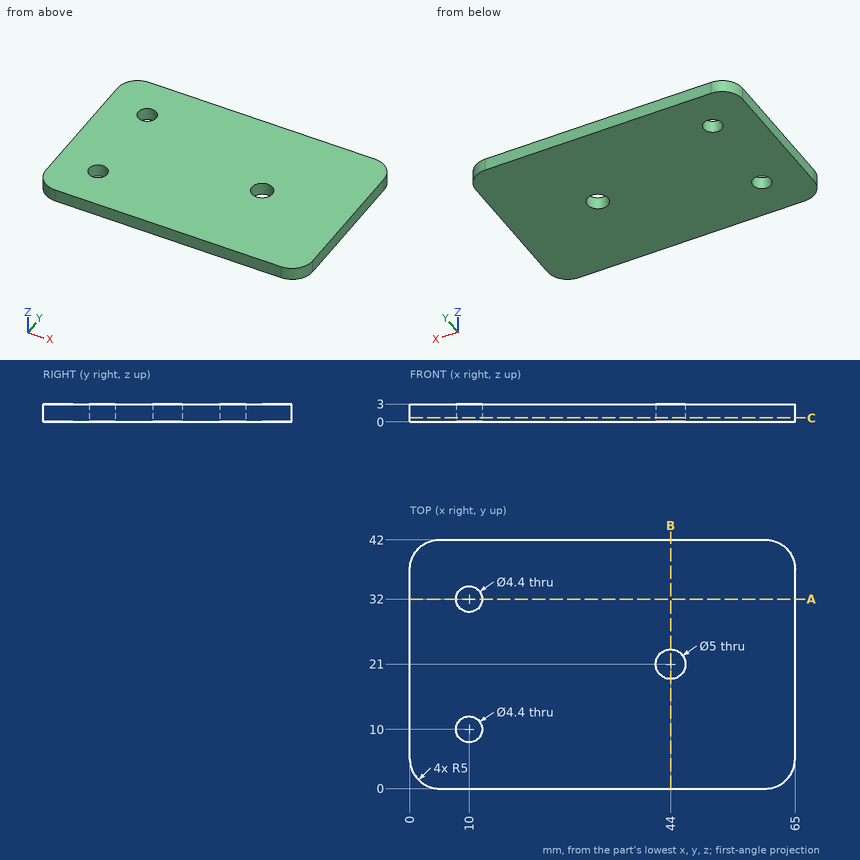
The figure shows three views and two pictorial views of one solid part (mm, origin at its lowest corner). Answer the questions. Give positions to 0.01 mm unless a question says otherwise; leave off trailing zeros. Loops run counter-clockwise (first coordinate to the right, second up) from the corner with the lowest first, then second, coordinate; pieces in that order, holes last. Notation, with made-up numbers: (64.25, 14) -> (87.25, 14) arc R31 ccw to (87.25, 38) -> close; hole circle Ø5 at (-2, 1). An arc over 180 degrees is marked (long way). Put each result on its own line as item: value. Start each with the question number.
Item 1: The part is cut by section C-C (z = 0.65). Give the vertices of the cut face in (x, y), then the cut area to 3 significant figures.
Item 2: The part is cut by section B-B (x = 44). Give the vertices of the cut face in (y, z).
Item 3: Find the intervals of material crossed by L1, parallel to Y at x = 10, z = 1.8; L2, parallel to X at y = 31, z = 2.65; L3, parallel to X at y = 23, z = 0.8, in increasing order. Write a range as [from, to].
Item 4: The part is cut by section A-A (y = 32). Give the vertices of the cut face in (x, z), then the cut area to 3 significant figures.
Answers below:
1. outline: (0, 5) arc R5 ccw to (5, 0) -> (60, 0) arc R5 ccw to (65, 5) -> (65, 37) arc R5 ccw to (60, 42) -> (5, 42) arc R5 ccw to (0, 37) -> close; hole circle Ø4.4 at (10, 10); hole circle Ø4.4 at (10, 32); hole circle Ø5 at (44, 21)
1. area: 2,660 mm2
2. outline: (0, 0) -> (18.5, 0) -> (18.5, 3) -> (0, 3) -> close; (23.5, 0) -> (42, 0) -> (42, 3) -> (23.5, 3) -> close
3. L1: [0, 7.8], [12.2, 29.8], [34.2, 42]
3. L2: [0, 8.04], [11.96, 65]
3. L3: [0, 42.5], [45.5, 65]
4. outline: (0, 0) -> (7.8, 0) -> (7.8, 3) -> (0, 3) -> close; (12.2, 0) -> (65, 0) -> (65, 3) -> (12.2, 3) -> close
4. area: 182 mm2
